```python
from build123d import *

# Parameters (mm, degrees)
F0_W      = 60
F0_H      = 40
F1_DEPTH  = 40
F2_W      = 60
F2_H      = 40
F3_DEPTH  = 30
F5_DEPTH  = 10.001
F6_W      = 25
F6_H      = 35
F7_DEPTH  = 10.001
F8_W      = 15
F8_H      = 15
F9_DEPTH  = 10.001
F10_R     = 5
F11_DEPTH = 10.001
F12_R     = 5
F13_DEPTH = 10.001
F14_R     = 15
F15_R     = 15


with BuildPart() as f1:
    # F0 (on Top) → F1 (new body)
    with BuildSketch(Plane.XY):
        with Locations((30, -20)):
            Rectangle(F0_W, F0_H)
    extrude(amount=F1_DEPTH)

    # F2 (on face) → F3 (cut)
    with BuildSketch(Plane.XY.offset(40)):
        with Locations((40, -30)):
            Rectangle(F2_W, F2_H)
    extrude(amount=-F3_DEPTH, mode=Mode.SUBTRACT)

    # F4 (on face) → F5 (cut, through all)
    with BuildSketch(Plane.YZ.offset(10)):
        Polygon((-30, 10), (-20, 40), (-20, 45), (-45, 45), (-45, 10), align=None)
    extrude(amount=-F5_DEPTH, mode=Mode.SUBTRACT)

    # F6 (on face) → F7 (cut, through all)
    with BuildSketch(Plane.XZ.offset(10)):
        with Locations((52.5, 27.5)):
            Rectangle(F6_W, F6_H)
    extrude(amount=-F7_DEPTH, mode=Mode.SUBTRACT)

    # F8 (on face) → F9 (cut, through all)
    with BuildSketch(Plane.XY.offset(10)):
        with Locations((57.5, -2.5)):
            Rectangle(F8_W, F8_H)
    extrude(amount=-F9_DEPTH, mode=Mode.SUBTRACT)

    # F10 (on face) → F11 (cut, through all)
    with BuildSketch(Plane.XY.offset(10)):
        with Locations((25, -25)):
            Circle(F10_R)
        with Locations((45, -25)):
            Circle(F10_R)
    extrude(amount=-F11_DEPTH, mode=Mode.SUBTRACT)

    # F12 (on face) → F13 (cut, through all)
    with BuildSketch(Plane.XZ.offset(10)):
        with Locations((25, 25)):
            Circle(F12_R)
    extrude(amount=-F13_DEPTH, mode=Mode.SUBTRACT)

    # F14
    f14_edges = [f1.edges().sort_by_distance(p)[0] for p in [
        (60, -40, 5),
    ]]
    fillet(f14_edges, radius=F14_R)

    # F15
    f15_edges = [f1.edges().sort_by_distance(p)[0] for p in [
        (40, -5, 40),
    ]]
    fillet(f15_edges, radius=F15_R)


solid = f1.part
```
Input: part model. Units: mm. Frame: model coordinates. A direction names the side the tool comes from. Give positions to 0.01 mm unless a question says otherwise; leave off trailing zeros. Order: outer loops, then holes, each group sorted by start corner. A loop starts at its lowest first (then second) coordinate and runs counter-clockwise, first axis right, second up. Notation, with made-up numbers: M 43.25,16.25 L 65.25,16.25 A32 ccw 65.25,46.25 Z; hole C 51,24.5 d8. An arc over 180 degrees is marked long. One line per question, with ' | ' between items. Start each with the question number.
1. Material intervals for probe 1 along Y at (x, z) = (25, 6); probe 2 along Y at (x, z) = (29, 30.5); probe 3 along X at (y, z) = (-28, 5.5), sorted ascending. Write a range as [from, to].
2. Section query C-C (x = 6). Return the cut outline in (y, z), and give its area (3 significant figures).
3. Section query A-A (y = -6.5). Return the cut outline in (x, z), and give its area (3 significant figures).
4. Pull-direction query (X, two-part tool) for faces 1 (the face through (60, -18, 5)), 2 (the face through (23.92, -5.07, 20.12)), 3 (the face through (30, -20, 0)); classes: released by +X, released by -X, zero draft, split by the parting line, or undercut.
5. Access query for faces 4 (the face through (0, -16, 15)), 5 (the face through (40, -5, 17)), 6 (the face through (55, -10, 5)), 7 (the face through (21, -10, 29)), 8 (the face through (22, -40, 5)). Directions: +Z, -Z, +X, -X, +Y, -Y. A direction counts if a zero-diameter tool reaches every point of the face in a straight line with its end or side. Return the directions, or none.
6. Section query D-D (y = -17). Return the cut outline in (x, z).
7. First-contact query: pin 1 Ø3 at (y, z) = (-3.5, 18.5) entering from +X; pin 2 Ø5 at (x, z) = (56, 3) entering from +Y; pin 3 Ø1.5 at (x, y) = (38, -34) entering from +Z. Flat tips, straight axial feed; report the tip coordinate or a pass-through.
8. Section query B-B (z = 5). Return the cut outline in (x, y), and give its area (3 significant figures).
Here are the results:
1) probe 1: [-40, -30], [-20, 0] | probe 2: [-10, 0] | probe 3: [0, 21], [29, 41], [49, 59.7]
2) outline: M -40,0 L 0,0 L 0,40 L -20,40 L -30,10 L -40,10 Z | area: 1,150 mm²
3) outline: M 0,0 L 50,0 L 50,10 L 40,10 L 40,25 A15 ccw 25,40 L 0,40 Z; hole C 25,25 d10 | area: 1,570 mm²
4) face 1: released by +X | face 2: undercut | face 3: zero draft
5) face 4: +Z, -Z, -X, +Y, -Y | face 5: +Z, +X, +Y, -Y | face 6: +Z, -Z, +X, +Y | face 7: +Z, +X, -Y | face 8: +Z, -Z, +X, -X, -Y
6) outline: M 0,0 L 60,0 L 60,10 L 10,10 L 10,40 L 0,40 Z
7) pin 1: x = 40 | pin 2: y = -10 | pin 3: z = 10
8) outline: M 0,-40 L 45,-40 A15 ccw 60,-25 L 60,-10 L 50,-10 L 50,0 L 0,0 Z; hole C 25,-25 d10; hole C 45,-25 d10 | area: 2,090 mm²
